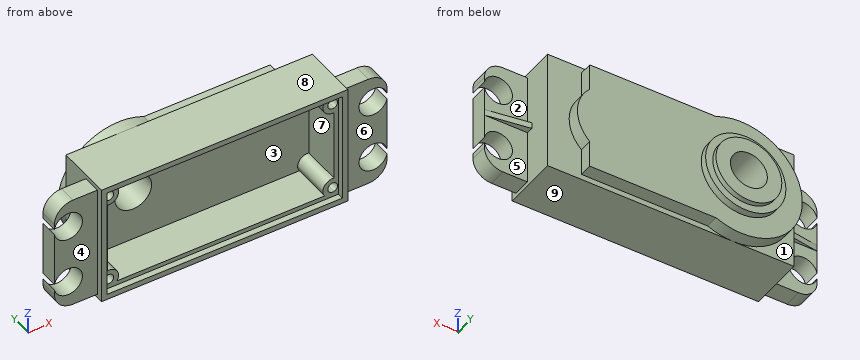
from build123d import *
from build123d.topology import SkipClean

# Parameters (mm, degrees)
SKETCH_1_W          = 40.05
SKETCH_1_H          = 19.8
EXTRUDE_1_DEPTH     = 9
SHELL_1_T           = -1.6
SKETCH_2_W          = 38.25
SKETCH_2_H          = 18
CUT_EXTRUDE_1_DEPTH = 1
EXTRUDE_2_DEPTH     = 2.1
SKETCH_4_R          = 6.525
EXTRUDE_3_DEPTH     = 1.1
SKETCH_5_R          = 5.35
EXTRUDE_4_DEPTH     = 0.8
CUT_EXTRUDE_START   = -5.6
SKETCH_6_R          = 3
CUT_EXTRUDE_2_DEPTH = 5.6
SKETCH_7_R          = 0.8
CUT_EXTRUDE_3_DEPTH = 14
SKETCH_8_R          = 1.6
SKETCH_8_R_2        = 0.8
EXTRUDE_5_DEPTH     = 6.4
SKETCH_9_R          = 0.8
EXTRUDE_6_DEPTH     = 1.6
EXTRUDE_7_DEPTH     = 7
CUT_EXTRUDE_4_DEPTH = 7
SKETCH_12_R         = 2.3
CUT_EXTRUDE_5_DEPTH = 7
EXTRUDE_8_DEPTH     = 7
SKETCH_16_R         = 2.3
CUT_EXTRUDE_6_DEPTH = 7
FILLET_1_R          = 3
CUT_EXTRUDE_7_DEPTH = 7


with BuildPart() as part:
    # Эскиз1 → Бобышка-Вытянуть1 (new body)
    with BuildSketch(Plane(origin=(0, 0, 0), x_dir=(1, 0, 0), z_dir=(0, 1, 0))):
        Rectangle(SKETCH_1_W, SKETCH_1_H)
    extrude(amount=EXTRUDE_1_DEPTH)

    # Оболочка1
    shell_1_openings = [part.faces().sort_by_distance(p)[0] for p in [
        (0, 0, 0),
    ]]
    offset(amount=SHELL_1_T, openings=shell_1_openings, kind=Kind.INTERSECTION)

    # Эскиз2 → Вырез-Вытянуть1 (cut)
    with BuildSketch(Plane.XZ):
        Rectangle(SKETCH_2_W, SKETCH_2_H)
    extrude(amount=-CUT_EXTRUDE_1_DEPTH, mode=Mode.SUBTRACT)

    # Эскиз3 → Бобышка-Вытянуть2 (add)
    with BuildSketch(Plane(origin=(0, 9, 0), x_dir=(1, 0, 0), z_dir=(0, 1, 0))):
        with BuildLine():
            Line((14.532872835, 4.640113908), (14.532872835, 9))
            Line((14.532872835, 9), (-6.000681875, 9))
            ThreePointArc((-6.000681875, 9), (-20.025, 0), (-6.000681875, -9))
            Line((-6.000681875, -9), (14.532872835, -9))
            Line((14.532872835, -9), (14.532872835, -4.640113908))
            ThreePointArc((14.532872835, -4.640113908), (16.525, 0), (14.532872835, 4.640113908))
        make_face()
    extrude(amount=EXTRUDE_2_DEPTH)

    # Эскиз4 → Бобышка-Вытянуть3 (add)
    with BuildSketch(Plane(origin=(0, 11.1, 0), x_dir=(1, 0, 0), z_dir=(0, 1, 0))):
        with Locations(Location((-10.125, 0, 0), (0, 0, 270))):
            Circle(SKETCH_4_R)
    extrude(amount=EXTRUDE_3_DEPTH)

    # Эскиз5 → Бобышка-Вытянуть4 (add)
    with BuildSketch(Plane(origin=(0, 12.2, 0), x_dir=(1, 0, 0), z_dir=(0, 1, 0))):
        with Locations(Location((-10.125, 0, 0), (0, 0, 270))):
            Circle(SKETCH_5_R)
    extrude(amount=EXTRUDE_4_DEPTH)

    # Эскиз6 → Вырез-Вытянуть2 (cut)
    with BuildSketch(Plane(origin=(0, 13, 0), x_dir=(1, 0, 0), z_dir=(0, 1, 0)).offset(CUT_EXTRUDE_START)):
        with Locations(Location((-10.125, 0, 0), (0, 0, 270))):
            Circle(SKETCH_6_R)
    extrude(amount=CUT_EXTRUDE_2_DEPTH, mode=Mode.SUBTRACT)

    # Эскиз7 → Вырез-Вытянуть3 (cut)
    with BuildSketch(Plane(origin=(0, 11.1, 0), x_dir=(1, 0, 0), z_dir=(0, 1, 0))):
        with Locations(Location((-18.2, 7.4, 0), (0, 0, 253.665177219))):
            Circle(SKETCH_7_R)
        with Locations(Location((18.2, 7.4, 0), (0, 0, 286.334822781))):
            Circle(SKETCH_7_R)
        with Locations(Location((18.2, -7.4, 0), (0, 0, 286.334822781))):
            Circle(SKETCH_7_R)
        with Locations(Location((-18.2, -7.4, 0), (0, 0, 253.665177219))):
            Circle(SKETCH_7_R)
    extrude(amount=-CUT_EXTRUDE_3_DEPTH, mode=Mode.SUBTRACT)

    # Эскиз8 → Бобышка-Вытянуть5 (add)
    # profile 1 of 4: a face of its own
    with SkipClean():  # the faces are left unmerged after this step: merging them gives an invalid solid
        with BuildSketch(Plane(origin=(0, 7.4, 0), x_dir=(-1, 0, 0), z_dir=(0, -1, 0))):
            with Locations((18.2, -7.4)):
                Circle(SKETCH_8_R)
            with Locations(Location((18.2, -7.4, 0), (0, 0, 270))):
                Circle(SKETCH_8_R_2, mode=Mode.SUBTRACT)
        # profile 2 of 4: a face of its own
        with BuildSketch(Plane(origin=(0, 7.4, 0), x_dir=(-1, 0, 0), z_dir=(0, -1, 0))):
            with Locations((18.2, 7.4)):
                Circle(SKETCH_8_R)
            with Locations(Location((18.2, 7.4, 0), (0, 0, 270))):
                Circle(SKETCH_8_R_2, mode=Mode.SUBTRACT)
        # profile 3 of 4: a face of its own
        with BuildSketch(Plane(origin=(0, 7.4, 0), x_dir=(-1, 0, 0), z_dir=(0, -1, 0))):
            with Locations((-18.2, 7.4)):
                Circle(SKETCH_8_R)
            with Locations(Location((-18.2, 7.4, 0), (0, 0, 270))):
                Circle(SKETCH_8_R_2, mode=Mode.SUBTRACT)
        # profile 4 of 4: a face of its own
        with BuildSketch(Plane(origin=(0, 7.4, 0), x_dir=(-1, 0, 0), z_dir=(0, -1, 0))):
            with Locations((-18.2, -7.4)):
                Circle(SKETCH_8_R)
            with Locations(Location((-18.2, -7.4, 0), (0, 0, 270))):
                Circle(SKETCH_8_R_2, mode=Mode.SUBTRACT)
        extrude(amount=EXTRUDE_5_DEPTH)

    # Эскиз9 → Бобышка-Вытянуть6 (add)
    with BuildSketch(Plane(origin=(0, 9, 0), x_dir=(1, 0, 0), z_dir=(0, 1, 0))):
        with Locations(Location((18.2, 7.4, 0), (0, 0, 270))):
            Circle(SKETCH_9_R)
        with Locations(Location((18.2, -7.4, 0), (0, 0, 270))):
            Circle(SKETCH_9_R)
        with Locations(Location((-18.2, -7.4, 0), (0, 0, 270))):
            Circle(SKETCH_9_R)
        with Locations(Location((-18.2, 7.4, 0), (0, 0, 270))):
            Circle(SKETCH_9_R)
    extrude(amount=-EXTRUDE_6_DEPTH)

    # Эскиз10 → Бобышка-Вытянуть7 (add)
    with BuildSketch(Plane(origin=(20.025, 0, 0), x_dir=(0, 0, -1), z_dir=(1, 0, 0))):
        Polygon((9.25, 1), (-9.25, 1), (-9.25, 3.9), (-0.5, 3.9), (-0.5, 5), (0.5, 5), (0.5, 3.9), (9.25, 3.9), align=None)
    extrude(amount=EXTRUDE_7_DEPTH)

    # Эскиз11 → Вырез-Вытянуть4 (cut)
    with BuildSketch(Plane.XY.offset(0.5)):
        Polygon((20.025, 5), (27.025, 3.9), (27.025, 5), align=None)
    extrude(amount=-CUT_EXTRUDE_4_DEPTH, mode=Mode.SUBTRACT)

    # Эскиз12 → Вырез-Вытянуть5 (cut)
    with BuildSketch(Plane(origin=(0, 3.9, 0), x_dir=(1, 0, 0), z_dir=(0, 1, 0))):
        with Locations((24.775, -4.9)):
            Circle(SKETCH_12_R)
        with Locations((24.775, 4.9)):
            Circle(SKETCH_12_R)
    extrude(amount=-CUT_EXTRUDE_5_DEPTH, mode=Mode.SUBTRACT)

    # Эскиз15 → Бобышка-Вытянуть8 (add)
    with BuildSketch(Plane.ZY.offset(20.025)):
        Polygon((-0.5, 3.9), (-9.25, 3.9), (-9.25, 1), (9.25, 1), (9.25, 3.9), (0.5, 3.9), (0.5, 5), (-0.5, 5), align=None)
    extrude(amount=EXTRUDE_8_DEPTH)

    # Эскиз16 → Вырез-Вытянуть6 (cut)
    with BuildSketch(Plane(origin=(0, 3.9, 0), x_dir=(1, 0, 0), z_dir=(0, 1, 0))):
        with Locations((-24.775, 4.9)):
            Circle(SKETCH_16_R)
        with Locations((-24.775, -4.9)):
            Circle(SKETCH_16_R)
    extrude(amount=-CUT_EXTRUDE_6_DEPTH, mode=Mode.SUBTRACT)

    # Скругление1
    fillet_1_edges = [part.edges().sort_by_distance(p)[0] for p in [
        (27.025, 2.45, -9.25),
        (27.025, 2.45, 9.25),
        (-27.025, 2.45, 9.25),
        (-27.025, 2.45, -9.25),
    ]]
    fillet(fillet_1_edges, radius=FILLET_1_R)

    # Эскиз17 → Вырез-Вытянуть7 (cut)
    with BuildSketch(Plane.XY.offset(0.5)):
        Polygon((-27.025, 3.9), (-20.025, 5), (-27.025, 5), align=None)
    extrude(amount=-CUT_EXTRUDE_7_DEPTH, mode=Mode.SUBTRACT)


solid = part.part
Can you work these out from the model? Positions are in its coordinate system, mm. Face numbers are marked on the shaded views. A direction names the side the tool comes from. Round coordinates to 2 decimals unless told otherwise and drop trailing zeros. Write each loop counter-clockwise with the first axis right and the second up, starting at its lowest first coordinate (ties: lowest second). Pieces come first, ordered by that corner, then holes. Notation, with made-up numbers: (30, -25) -> (74, -25) arc R12 cw to (74, -20) -> close; hole circle Ø10 at (-19, -40). An arc over 180 degrees is marked (long way). Use one line per item in the form item = value. Start each with the question number.
Q1. Which directions (+Z, -Z, +X, -X, +Y, -Y) give clear straight access to the entire face, cutting with the end or side of a thin tool? Please do the marked faces 1, 2, 3, 4 and 5.
Q2. We'd pull the mould along Z, two halves only. Please class the marked faces 6, 7, 8 and 9: +Z half, -Z half, draft (parallel to the pull), parting line (faces both ways), or undercut.
Q3. Imagine slicing it at B-B (x = 23.5). Please give me the cut outline in (y, z), then the cut area to 3 significant figures.
Q4. Imagine slicing it at C-C (z = -3.75). Count the separate pieces of the cut face and the enclosed holes in it, then the cut area to 3 significant figures.
Q5. If I drill on probe 1 along Z at (x, y) = (18.2, 5.5); probe 2 along X at (y, z) = (6.25, -7.4) (3 decimals); probe 3 along X at (y, z) = (7.25, 5.5) (3 decimals), over which ranges is the centre line in solid material (lowest first)? Write a range as [from, to].
Q6. I'm going to push flat-ended pins straight in: P1, Ø4, axis at x = -17, z = 4, coming from the -Y side; P2, Ø2, axis at x = 22, z = 5.5, coming from the +Y side; P3, Ø1.5, axis at y = 10.5, z = -1, coming from the -X side. Where does each tip first touch, or does it pass through?
Q7. Imagine slicing it at A-A (y = 5.5). Please give me the cut outline in (x, z) (3 decimals).
Worked out:
q1.face_1 = -Z, -X, +Y
q1.face_2 = +Z, +X, +Y
q1.face_3 = -Y
q1.face_4 = +Z, -Z, -X, -Y
q1.face_5 = -Z, +X, +Y
q2.face_6 = draft
q2.face_7 = undercut
q2.face_8 = +Z half
q2.face_9 = -Z half
q3.outline = (1, -9.25) -> (3.9, -9.25) -> (3.9, -6.81) -> (1, -6.81) -> close; (1, -2.99) -> (3.9, -2.99) -> (3.9, -0.5) -> (4.45, -0.5) -> (4.45, 0.5) -> (3.9, 0.5) -> (3.9, 2.99) -> (1, 2.99) -> close; (1, 6.81) -> (3.9, 6.81) -> (3.9, 9.25) -> (1, 9.25) -> close
q3.area = 32.0 mm^2
q4.separate_pieces = 3
q4.enclosed_holes = 0
q4.area = 194 mm^2
q5.probe_1 = [-9.9, -8.2], [-6.6, -5.8], [5.8, 6.6], [8.2, 9.9]
q5.probe_2 = [-20.025, -19], [-17.4, -16.6], [16.6, 17.4], [19, 20.025]
q5.probe_3 = [-20.025, -18.425], [18.425, 20.025]
q6.P1 = 1
q6.P2 = 3.9
q6.P3 = -20.02
q7.outline = (-20.025, -9.9) -> (20.025, -9.9) -> (20.025, 9.9) -> (-20.025, 9.9) -> close; hole circle Ø1.6 at (-18.2, -7.4); hole circle Ø1.6 at (-18.2, 7.4); hole (-18.425, -5.816) arc R1.6 cw to (-16.877, -8.3) -> (16.877, -8.3) arc R1.6 cw to (18.425, -5.816) -> (18.425, 5.816) arc R1.6 cw to (16.877, 8.3) -> (-16.877, 8.3) arc R1.6 cw to (-18.425, 5.816) -> close; hole circle Ø1.6 at (18.2, -7.4); hole circle Ø1.6 at (18.2, 7.4)
